Could you check a few things on this model? Use its own coordinates, in mm. A direction names the side the tool comes from. Round coordinates to 2 decimals unless told otherwise and drop trailing zeros. Write each loop counter-clockwise with the first axis right and the second up, starting at its lowest first coordinate (ties: lowest second). Pieces come first, ordered by that corner, then holes. Notation, with made-up numbers: (60.25, 85) -> (109.25, 85) arc R26 ccw to (109.25, 101) -> close; hole circle Ø3 at (10.25, -20.5). An arc over 180 degrees is marked (long way). Answer in a Markdown table with one row per item.
from build123d import *

# Parameters (mm, degrees)
F1_DEPTH = 2
F2_R     = 2
F3_DEPTH = 10
F4_SIZE  = 1
F5_R     = 1.5
F6_DEPTH = 3
F9_SIZE  = 0.5


with BuildPart() as f1:
    # F0 (on Top) → F1 (new body)
    with BuildSketch(Plane.XY):
        Polygon((4.5, -2.5980762114), (4.5, 2.5980762114), (0, 5.1961524227), (-4.5, 2.5980762114), (-4.5, -2.5980762114), (0, -5.1961524227), align=None)
    extrude(amount=F1_DEPTH)

    # F2 (on face) → F3 (join)
    with BuildSketch(Plane(origin=(0, 0, 0), x_dir=(1, 0, 0), z_dir=(0, 0, -1))):
        Circle(F2_R)
    extrude(amount=F3_DEPTH)

    # F4
    f4_edges = [f1.edges().sort_by_distance(p)[0] for p in [
        (-2, 0, -10),
    ]]
    chamfer(f4_edges, length=F4_SIZE)

    # F5 (on face) → F6 (join)
    with BuildSketch(Plane.XY.offset(2)):
        Circle(F5_R)
    extrude(amount=F6_DEPTH)

    # F7 (on Front) → F8 (revolve)
    with BuildSketch(Plane.XZ):
        with BuildLine():
            Line((1.5, 5), (1.5, 4.6771243445))
            ThreePointArc((1.5, 4.6771243445), (1.8228756555, 6.8228756555), (0, 8))
            Line((0, 8), (0, 5))
            Line((0, 5), (1.5, 5))
        make_face()
    revolve(axis=Axis((0, 0, 2), (0, 0, 1)))

    # F9
    f9_edges = [f1.edges().sort_by_distance(p)[0] for p in [
        (2.25, -3.897114, 2),
        (4.5, 0, 2),
        (2.25, 3.897114, 2),
        (-2.25, 3.897114, 2),
        (-2.25, -3.897114, 2),
        (-4.5, 0, 2),
        (-1.5, 0, 2),
    ]]
    chamfer(f9_edges, length=F9_SIZE)


solid = f1.part
1) Imagine slicing it at D-D, the plane y = -3.25. Please give me the cut outline in (x, z), plus the area to 3 significant figures.
Findings:
| item | result |
|---|---|
| outline | (-3.37, 0) -> (3.37, 0) -> (3.37, 1.5) -> (2.37, 2) -> (-2.37, 2) -> (-3.37, 1.5) -> close |
| area | 13.0 mm^2 |
2) Imagine slicing it at C-C, the plane z = -7.5. Please give me the cut outline in (x, y), plus the area to 3 significant figures.
Findings:
| item | result |
|---|---|
| outline | circle Ø4 at (0, 0) |
| area | 12.6 mm^2 |
3) Imagine slicing it at A-A, the plane y = 0. Please give me the cut outline in (x, z).
Findings:
| item | result |
|---|---|
| outline | (-4.5, 0) -> (-2, 0) -> (-2, -9) -> (-1, -10) -> (1, -10) -> (2, -9) -> (2, 0) -> (4.5, 0) -> (4.5, 1.5) -> (4, 2) -> (2, 2) -> (1.5, 2.5) -> (1.5, 4.68) arc R2 ccw (long way) to (-1.5, 4.68) -> (-1.5, 2.5) -> (-2, 2) -> (-4, 2) -> (-4.5, 1.5) -> close |
4) Imagine slicing it at B-B, the plane x = -3.25. Please give me the cut outline in (y, z), plus the area to 3 significant figures.
Findings:
| item | result |
|---|---|
| outline | (-3.32, 0) -> (3.32, 0) -> (3.32, 1.5) -> (2.74, 2) -> (-2.74, 2) -> (-3.32, 1.5) -> close |
| area | 13.0 mm^2 |
5) For pin 1 (3 mm diameter, centred on x = 2, z = -3, fed in from +Y); pin 2 (2 mm diameter, centred on x = 1.5, y = -4, fed in from -Z); pin 3 (4 mm diameter, centred on x = -3.5, z = -4.5, fed in from -Y), each with a flat end and sliding along its axis, tell me the tip position at first contact or that it passes through.
Findings:
| item | result |
|---|---|
| pin 1 | stops at y = 1.94 |
| pin 2 | stops at z = 0 |
| pin 3 | stops at y = -1.32 |
6) Thinking about a two-plate mould opening in Z: for faces 4 (the face through (2.158, 3.665, 1.747)), 5 (the face through (-4.5, 0, 1)), 6 (the face through (0, 0, -10)), 7 (the face through (-1.5, 0.07, 3.57)), which applies, +Z half, -Z half, draft (parallel to the pull), parting line (faces both ways), or undercut?
Findings:
| item | result |
|---|---|
| face 4 | +Z half |
| face 5 | draft |
| face 6 | -Z half |
| face 7 | undercut |
7) For faces 1 (the face through (-0.1, -2.2, 0)), 2 (the face through (-2, -1, 2)), 3 (the face through (-2.28, -3.88, 0.74)), which set-ups out of +Z, -Z, +X, -X, +Y, -Y let a thin tool reach every point of the face, with its end or its side?
Findings:
| item | result |
|---|---|
| face 1 | -Z |
| face 2 | +Z |
| face 3 | +Z, -Z, -X, -Y |
8) Please list where these lines run through material, in increasing order: line 1 (Z direction, x = 1.75, y = -3.25); line 2 (Z direction, x = -1, y = -1.5); line 3 (X direction, y = -1, z = -1.75).
Findings:
| item | result |
|---|---|
| line 1 | z = 0 to 2 |
| line 2 | z = -9.2 to 2.2, 5.13 to 6.87 |
| line 3 | x = -1.73 to 1.73 |
